Can you work these out from the model? Positions are in its coordinate system, mm. A direction names the side the tool comes from. Round coordinates to 2 decimals unless told otherwise and drop trailing zeros. Loops run counter-clockwise (first coordinate to the right, second up) from the corner with the lowest first, then second, coordinate; pieces in that order, holes last.
```python
from build123d import *

# Parameters (mm, degrees)
SKETCH4_W           = 72
SKETCH4_H           = 72
SKETCH4_R           = 3
SKETCH4_R_2         = 2.5
SKETCH4_R_3         = 2.35
BOSS_EXTRUDE2_DEPTH = 5
SKETCH5_W           = 10.4
SKETCH5_H           = 1.2
SKETCH5_W_2         = 1.2
SKETCH5_H_2         = 10.4
CUT_EXTRUDE1_DEPTH  = 2
CUT_EXTRUDE2_DEPTH  = 2.1
FILLET1_R           = 10
SKETCH7_R           = 1.75
CUT_EXTRUDE3_DEPTH  = 5
SKETCH8_R           = 1.75
CUT_EXTRUDE4_DEPTH  = 5


with BuildPart() as part:
    # Sketch3 → Revolve1 (revolve)
    with BuildSketch(Plane.XY, mode=Mode.PRIVATE) as revolve1_sk:
        with BuildLine():
            Line((0, 0), (2.7, 0))
            Line((2.7, 0), (2.233206222, 1.282505364))
            ThreePointArc((2.233206222, 1.282505364), (1.26348021, 0.413869711), (0, 0.1))
            Line((0, 0.1), (0, 0))
        make_face()
    revolve(revolve1_sk.sketch.rotate(Axis((0, 0.1, 0), (0, -1, 0)), 90), axis=Axis((0, 0.1, 0), (0, -1, 0)))

    # Sketch4 → Boss-Extrude2 (add)
    with BuildSketch(Plane.XZ):
        Rectangle(SKETCH4_W, SKETCH4_H)
        with Locations(Location((23, 0, 0), (0, 0, 270))):
            Circle(SKETCH4_R, mode=Mode.SUBTRACT)
        with Locations(Location((0, 23, 0), (0, 0, 270))):
            Circle(SKETCH4_R, mode=Mode.SUBTRACT)
        with Locations(Location((-15, -15, 0), (0, 0, 270))):
            Circle(SKETCH4_R_2, mode=Mode.SUBTRACT)
        with Locations(Location((0, 31, 0), (0, 0, 270))):
            Circle(SKETCH4_R_3, mode=Mode.SUBTRACT)
        with Locations(Location((31, 0, 0), (0, 0, 270))):
            Circle(SKETCH4_R_3, mode=Mode.SUBTRACT)
    extrude(amount=BOSS_EXTRUDE2_DEPTH)

    # Sketch5 → Cut-Extrude1 (cut)
    with BuildSketch(Plane.XZ.offset(5)):
        with Locations((0, 23)):
            Rectangle(SKETCH5_W, SKETCH5_H)
        with Locations((23, 0)):
            Rectangle(SKETCH5_W_2, SKETCH5_H_2)
        Polygon((-18.252691193, -10.898780669), (-10.898780669, -18.252691193), (-11.747308807, -19.101219331), (-19.101219331, -11.747308807), align=None)
    extrude(amount=-CUT_EXTRUDE1_DEPTH, mode=Mode.SUBTRACT)

    # Sketch6 → Cut-Extrude2 (cut)
    with BuildSketch(Plane(origin=(0, 0, 0), x_dir=(1, 0, 0), z_dir=(0, 1, 0))):
        Polygon((1.789785834, -27.9), (-1.789785834, -27.9), (-3.579571669, -31), (-1.789785834, -34.1), (1.789785834, -34.1), (3.579571669, -31), align=None)
        Polygon((34.1, 1.789785834), (31, 3.579571669), (27.9, 1.789785834), (27.9, -1.789785834), (31, -3.579571669), (34.1, -1.789785834), align=None)
    extrude(amount=-CUT_EXTRUDE2_DEPTH, mode=Mode.SUBTRACT)

    # Fillet1
    fillet1_edges = [part.edges().sort_by_distance(p)[0] for p in [
        (36, -2.5, -36),
        (36, -2.5, 36),
        (-36, -2.5, 36),
        (-36, -2.5, -36),
    ]]
    fillet(fillet1_edges, radius=FILLET1_R)

    # Sketch7 → Cut-Extrude3 (cut)
    with BuildSketch(Plane.XZ.offset(5)):
        with Locations(Location((22.26, 25.07, 0), (0, 0, 270))):
            Circle(SKETCH7_R)
    extrude(amount=-CUT_EXTRUDE3_DEPTH, mode=Mode.SUBTRACT)

    # Sketch8 → Cut-Extrude4 (cut)
    with BuildSketch(Plane.XZ.offset(5)):
        with Locations(Location((-27.74, -24.34, 0), (0, 0, 270))):
            Circle(SKETCH8_R)
    extrude(amount=-CUT_EXTRUDE4_DEPTH, mode=Mode.SUBTRACT)


solid = part.part
```
(1) If I drill on line 1 (X direction, y = -3.5, z = 0); line 2 (X direction, y = -3.15, z = -15), over which ranges is the centre line in solid material (lowest first)?
(2) Suppose I cut it at B-B (z = -24.34). Write out the boundary of the cut face in (x, y), then the cut area to 4 significant figures.
(3) For pin 1 (7 mm diameter, centred on x = -1.5, z = 31.5, fed in from +Y), with a flat end and sliding along its axis, tell me the tip position at first contact or that it passes through.
(4) Suppose I cut it at A-A (y = -1.25). Write out the boundary of the cut face in (x, z), then the cut area to 3 significant figures.
(5) We'd pull the mould along Z, two halves only. Please class faces 1 (the cylindrical face through (32.99, -2.54, 33.15)), 2 (the flat face through (-36, -2, 0)), 3 (the flat face through (2, -2.1, 29)): released by +Z, released by -Z, zero draft, split by the parting line, or undercut.
(6) Which directions (+Z, -Z, +X, -X, +Y, -Y) give clear straight access to the entire face, cutting with the end or side of a thin tool? Please do faces 4 (the cylindrical face through (-2.93, -2.46, 23.65)), 5 (the flat face through (4, -4, 22.4)), 6 (the flat face through (27.9, -1, 0)).
(7) Suppose I cut it at D-D (x = 0). Write out the boundary of the cut face in (y, z), then the cut area to 3 significant figures.
(8) Suppose I cut it at C-C (x = -15). Write out the boundary of the cut face in (y, z), then the cut area to 3 significant figures.
Check result:
1. line 1: x = -36 to 20, 26 to 28.65, 33.35 to 36
1. line 2: x = -36 to -17.5, -12.5 to 36
2. outline: (-36, -5) - (-29.49, -5) - (-29.49, 0) - (-36, 0) - close; (-25.99, -5) - (36, -5) - (36, 0) - (-25.99, 0) - close
2. area: 342.5 mm2
3. pin 1: stops at y = 0
4. outline: (-36, -26) arc R10 ccw to (-26, -36) - (26, -36) arc R10 ccw to (36, -26) - (36, 26) arc R10 ccw to (26, 36) - (-26, 36) arc R10 ccw to (-36, 26) - close; hole circle Ø3.5 at (-27.74, -24.34); hole circle Ø5 at (-15, -15); hole (-3.58, 31) - (-1.79, 27.9) - (1.79, 27.9) - (3.58, 31) - (1.79, 34.1) - (-1.79, 34.1) - close; hole circle Ø6 at (0, 23); hole circle Ø6 at (23, 0); hole circle Ø3.5 at (22.26, 25.07); hole (27.9, -1.79) - (31, -3.58) - (34.1, -1.79) - (34.1, 1.79) - (31, 3.58) - (27.9, 1.79) - close
4. area: 4,940 mm2
5. face 1: released by +Z
5. face 2: zero draft
5. face 3: undercut
6. face 4: +Y, -Y
6. face 5: -Y
6. face 6: +Y
7. outline: (-5, -36) - (0, -36) - (0, -2.7) - (1.28, -2.23) arc R2.7 cw to (1.28, 2.23) - (0, 2.7) - (0, 20) - (-5, 20) - close; (-5, 26) - (0, 26) - (0, 27.9) - (-2.1, 27.9) - (-2.1, 28.65) - (-5, 28.65) - close; (-5, 33.35) - (-2.1, 33.35) - (-2.1, 34.1) - (0, 34.1) - (0, 36) - (-5, 36) - close
7. area: 306 mm2
8. outline: (-5, -36) - (0, -36) - (0, -17.5) - (-5, -17.5) - close; (-5, -12.5) - (0, -12.5) - (0, 36) - (-5, 36) - close
8. area: 335 mm2
